```python
from build123d import *

# Parameters (mm, degrees)
F0_W     = 15
F0_H     = 15
F0_W_2   = 20
F0_H_2   = 20
F1_DEPTH = 3


with BuildPart() as f1:
    # F0 (on Top) → F1 (new body)
    with BuildSketch(Plane.XY):
        Polygon((-30, 0), (-15, 0), (-15, 15), (0, 15), (0, 30), (-30, 30), align=None)
        with Locations((-7.5, 7.5)):
            Rectangle(F0_W, F0_H)
        with Locations((10, 7.5)):
            Rectangle(F0_W_2, F0_H)
        with Locations((-7.5, -10)):
            Rectangle(F0_W, F0_H_2)
        Polygon((0, 30), (0, 15), (20, 15), align=None)
        Polygon((-15, -20), (-15, 0), (-30, 0), align=None)
    extrude(amount=F1_DEPTH)


solid = f1.part
```
For this review, take the finished solid that the model builds, in its own axes (mm). A direction names the side the tool comes from. Give positions to 0.01 mm unless a question says otherwise; leave off trailing zeros. Write each loop counter-clockwise with the first axis right and the second up, starting at its lowest first coordinate (ties: lowest second). Pieces come first, ordered by that corner, then holes. Notation, with made-up numbers: M 84.5,16 L 133.5,16 A30 cw 133.5,46 Z; hole C -37.5,-22.75 d8. An arc over 180 degrees is marked long. Answer as a JSON object with one key per item and string values. Group by question number.
Item 1: Consider section C-C on x = -26.5. Write out the cut boundary in (y, z), plus the area to 3 significant figures.
Item 2: For pin 1 Ø0.9 at (x, z) = (10.5, 1.5) entering from -Y; pin 2 Ø1.5 at (y, z) = (-2.5, 2.5) entering from +X; pin 3 Ø2 at (x, y) = (-11, 4) entering from -Z, all flat-tipped, find the tip position at first contact; note any pin that passes through.
Item 3: Consider section A-A on z = 1.2. Write out the cut boundary in (x, y).
Item 4: Tool access review of faces 1 (the flat face through (-11, 11, 3)), 2 (the flat face through (10, 0, 1)): name each direction out of +Z, -Z, +X, -X, +Y, -Y from which nothing blocks a thin tool from reaching the whole face with its end or side.
Item 5: Consider section B-B on y = -7. Write out the cut boundary in (x, z), plus the area to 4 significant figures.
Item 6: For probe 1 along Y at (x, z) = (17.5, 2.6) (3 decimals); probe 2 along Y at (x, z) = (10, 0.5); probe 3 along X at (y, z) = (18, 1), list the stretches that pass through material, from the lowest coordinate up. Write a range as [from, to].
Check result:
{
 "1": {"outline": "M -4.67,0 L 30,0 L 30,3 L -4.67,3 Z", "area": "104 mm^2"},
 "2": {"pin 1": "stops at y = 0", "pin 2": "stops at x = 0", "pin 3": "stops at z = 0"},
 "3": {"outline": "M -30,0 L -15,-20 L 0,-20 L 0,0 L 20,0 L 20,15 L 0,30 L -30,30 Z"},
 "4": {"face 1": "+Z, +X, -X, +Y, -Y", "face 2": "+Z, -Z, +X, -Y"},
 "5": {"outline": "M -24.75,0 L 0,0 L 0,3 L -24.75,3 Z", "area": "74.25 mm^2"},
 "6": {"probe 1": "y = [0, 16.875]", "probe 2": "y = [0, 22.5]", "probe 3": "x = [-30, 16]"}
}
